Input: part model. Units: mm. Frame: model coordinates. A direction names the side the tool comes from. Round coordinates to 2 decimals unless told otherwise and drop trailing zeros. Order: outer loops, then holes, each group sorted by start corner. A loop starts at its lowest first (then second) coordinate and runs counter-clockwise, first axis right, second up. Notation, with made-up numbers: (3.5, -11.5) -> (39.5, -11.5) arc R32 ccw to (39.5, 14.5) -> close; hole circle Ø5 at (83, -39). An arc over 180 degrees is marked (long way). Answer as CSV lines item,"result". Start each with the question number.
1) Section query C-C, the plane y = 0.5. Output: boundary loops of the cut face in (x, z), and give its area (3 significant figures).
2) Line query: L1, parallel to X at y = 1.5, z = -10; L2, parallel to Z at x = -13, y = 4.5; L3, parallel to Z at x = -3.5, y = 5.75. Output: solid intervals per line, ascending.
3) Access query for faces 3 (the face through (4, 0, -14)), 4 (the face through (1, 3, 15)). Directions: +Z, -Z, +X, -X, +Y, -Y. A direction counts if a zero-diameter tool reaches every point of the face in a straight line with its end or side. Return the directions, or none.
4) First-contact query: P1, Ø3, axis at y = 1, z = 11.5, coming from the +X side; P2, Ø8, axis at x = -9, z = 6.5, coming from the -Y side; P3, Ø1.5, axis at y = 3, z = -2, coming from the -X side; P4, Ø1, axis at y = 1, z = -3, coming from the +X side. Flat tips, straight axial feed; report the tip coordinate or a pass-through.
5) Section query A-A, the plane z = 0. Output: boundary loops of the cut face in (x, y), and give its area (3 significant figures).
6) Mould query, pull axis X, two halves, no side actions, for faces 1 (the face through (14, 7.5, -5)), 2 (the face through (-1, 3, 15)). Classes: +X half, -X half, draft (parallel to the pull), parting line (faces both ways), or undercut.
7) Section query B-B, the plane y = 5.75. Output: boundary loops of the cut face in (x, z).
```python
from build123d import *

# Parameters (mm, degrees)
ESQUISSE2_W             = 2
ESQUISSE2_H             = 7.5
ENL_V_MAT_EXTRU_4_DEPTH = 18


with BuildPart() as part:
    # Esquisse1 → Révolution1 (revolve)
    with BuildSketch(Plane.XY, mode=Mode.PRIVATE) as r_volution1_sk:
        Polygon((14.25, 0), (14.25, 7.5), (15.268488567, 7.5), (17, 0), align=None)
    revolve(r_volution1_sk.sketch.rotate(Axis((0, -11.232892416, 0), (0, 1, 0)), 90), axis=Axis((0, -11.232892416, 0), (0, 1, 0)))  # turned: the seam where the file's is

    # Esquisse2 → Enlèv. mat.-Extru.4 (cut, through all)
    with BuildSketch(Plane.XY):
        with Locations((0, 3.75)):
            Rectangle(ESQUISSE2_W, ESQUISSE2_H)
    extrude(amount=ENL_V_MAT_EXTRU_4_DEPTH, mode=Mode.SUBTRACT)


solid = part.part
```
Findings:
1,outline,"(-1, 14.21) -> (-1, 16.85) arc R16.88 ccw (long way) to (1, 16.85) -> (1, 14.21) arc R14.25 cw (long way) to start"
1,area,"252 mm^2"
2,L1,"x = -13.32 to -10.15, 10.15 to 13.32"
2,L2,"z = -9.26 to -5.84, 5.84 to 9.26"
2,L3,"z = -15.28 to -13.81, 13.81 to 15.28"
3,face 3,"+Z, -Z, +X, -X, -Y"
3,face 4,"+Z, +Y, -Y"
4,P1,"stops at x = 13.54"
4,P2,"stops at y = 0"
4,P3,"stops at x = -16.38"
4,P4,"stops at x = 16.64"
5,outline,"(-17, 0) -> (-14.25, 0) -> (-14.25, 7.5) -> (-15.27, 7.5) -> close; (14.25, 0) -> (17, 0) -> (15.27, 7.5) -> (14.25, 7.5) -> close"
5,area,"28.3 mm^2"
6,face 1,"draft"
6,face 2,"undercut"
7,outline,"(-1, 14.21) -> (-1, 15.64) arc R15.67 ccw (long way) to (1, 15.64) -> (1, 14.21) arc R14.25 cw (long way) to start"
